Work out the finished part from the listing and answer in its coordinate system (mm). Give positions to 0.01 mm unless a question says otherwise; leave off trailing zeros. Write each loop counter-clockwise with the first axis right and the second up, starting at its lowest first coordinate (ties: lowest second). Pieces come first, ordered by that corner, then holes. Notation, with made-up numbers: (-16, 48) -> (-10, 48) arc R7 cw to (-10, 55) -> close; hole circle Ø8 at (62, 86.25). An arc over 180 degrees is marked (long way). Use a Markdown table: item, result. Add a question column.
Q1. Each of these flat-tipped pins is pushed along its axis until it touches: pin 1 Ø4 at (x, y) = (-15.14, -230.12) entering from -Z; pin 2 Ø10 at (x, y) = (84.5, -95) entering from +Z. Where does it stop, or does it pass through?
Q2. Consider line 1 (X direction, y = -162, z = 0.9); line 2 (Y direction, x = 116, z = 1.55). Determine where each line is inside the solid, lowest interval first.
Q3. Section B-B, the plane x = 73.5 is taken. State how many separate pieces and enclosed holes the cut face has, plus the area to 3 significant figures.
Q4. Section A-A, the plane y = -100 is taken. Give the vertices of the cut face in (x, z), plus the area to 3 significant figures.
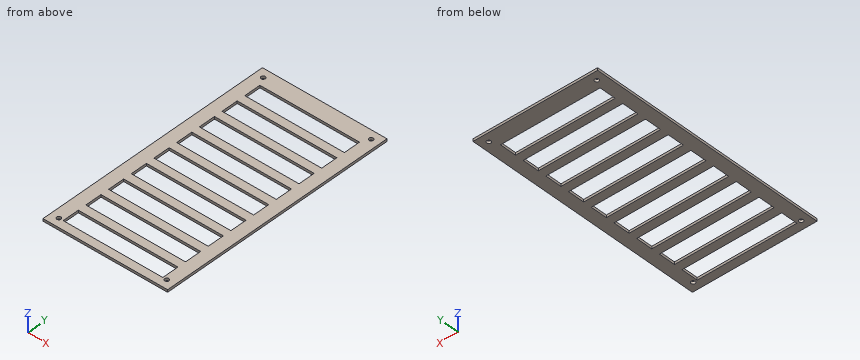
from build123d import *

# Parameters (mm, degrees)
SKETCH_1_W             = 150
SKETCH_1_H             = 290
EXTRUDE_1_DEPTH        = 3
SKETCH_2_R             = 2.5
CUT_EXTRUDE_1_DEPTH    = 3
SKETCH_3_W             = 120
SKETCH_3_H             = 20
CUT_EXTRUDE_2_DEPTH    = 3
PATTERN_LINEAR_1_COUNT = 9
PATTERN_LINEAR_1_PITCH = 30


with BuildPart() as part:
    # 草图1 → 凸台-拉伸1 (new body)
    with BuildSketch(Plane.XY):
        with Locations((49.855231415, -95.12154255)):
            Rectangle(SKETCH_1_W, SKETCH_1_H)
    extrude(amount=EXTRUDE_1_DEPTH)

    # 草图2 → 切除-拉伸1 (cut)
    with BuildSketch(Plane.XY.offset(3)):
        with Locations((114.855231415, 39.87845745)):
            Circle(SKETCH_2_R)
        with Locations((114.855231415, -230.12154255)):
            Circle(SKETCH_2_R)
        with Locations((-15.144768585, 39.87845745)):
            Circle(SKETCH_2_R)
        with Locations((-15.144768585, -230.12154255)):
            Circle(SKETCH_2_R)
    extrude(amount=-CUT_EXTRUDE_1_DEPTH, mode=Mode.SUBTRACT)

    # 草图3 → 切除-拉伸2 (cut)
    with BuildSketch(Plane.XY.offset(3)):
        with Locations((50.020248586, 19.87845745)):
            Rectangle(SKETCH_3_W, SKETCH_3_H)
    cut_extrude_2 = extrude(amount=-CUT_EXTRUDE_2_DEPTH, mode=Mode.SUBTRACT)

    # 阵列(线性)1: 切除-拉伸2 ×9
    with Locations(*[(0, -i * PATTERN_LINEAR_1_PITCH, 0) for i in range(1, PATTERN_LINEAR_1_COUNT)]):
        add(cut_extrude_2, mode=Mode.SUBTRACT)


solid = part.part
Result set:
| question | item | result |
|---|---|---|
| 1 | pin 1 | passes through |
| 1 | pin 2 | stops at z = 3 |
| 2 | line 1 | x = -25.14 to -9.98, 110.02 to 124.86 |
| 2 | line 2 | y = -240.12 to -232.34, -227.9 to 37.66, 42.1 to 49.88 |
| 3 | separate pieces | 10 |
| 3 | enclosed holes | 0 |
| 3 | area | 330 mm2 |
| 4 | outline | (-25.14, 0) -> (-9.98, 0) -> (-9.98, 3) -> (-25.14, 3) -> close; (110.02, 0) -> (124.86, 0) -> (124.86, 3) -> (110.02, 3) -> close |
| 4 | area | 90.0 mm2 |
